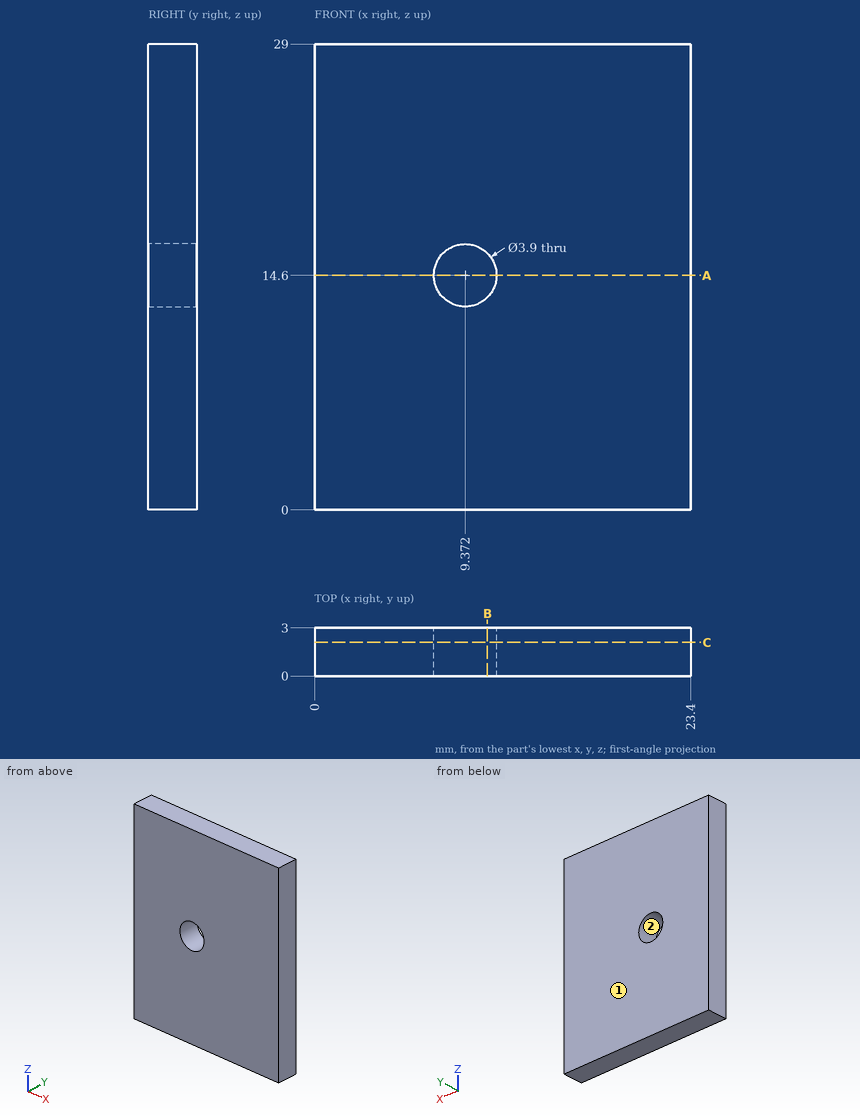
Here's the drawing with two shaded views (mm, measured from the low corner). I have some questions. Give positions to 0.01 mm unless a question says otherwise; leave off trailing zeros. Order: outer loops, then holes, each group sorted by start corner. A loop starts at its lowest first (then second) coordinate and runs counter-clockwise, first axis right, second up.
Q1. If I drill on line 1 along X through (y, z) = (1.95, 14.6); line 2 along X through (y, z) = (1.2, 13); line 3 along Z through (x, y) = (8.25, 0.7) (1 decimal), over which ranges is the centre line in solid material (lowest first)?
Q2. We'd pull the mould along Z, two halves only. Please class the marked faces 1 and 2: +Z half, -Z half, draft (parallel to the pull), parting line (faces both ways), or undercut.
Q3. Suppose I cut it at A-A, the plane z = 14.6. Write out the boundary of the cut face in (x, y).
Q4. Suppose I cut it at B-B, the plane x = 10.75. Write out the boundary of the cut face in (y, z), and give its area (3 significant figures).
Q5. Suppose I cut it at C-C, the plane y = 2.1. Write out the boundary of the cut face in (x, z).
Q6. I'm going to push flat-ended pins straight in: P1, Ø4, axis at x = 5.5, z = 7, coming from the -Y side; P2, Ø3.5, axis at x = 9.37, z = 14.6, coming from the -Y side. Where does each tip first touch, or does it pass through?
Solution:
1. line 1: x = 0 to 7.42, 11.32 to 23.4
1. line 2: x = 0 to 8.26, 10.49 to 23.4
1. line 3: z = 0 to 13, 16.2 to 29
2. face 1: draft
2. face 2: undercut
3. outline: (0, 0) - (7.42, 0) - (7.42, 3) - (0, 3) - close; (11.32, 0) - (23.4, 0) - (23.4, 3) - (11.32, 3) - close
4. outline: (0, 0) - (3, 0) - (3, 13.22) - (0, 13.22) - close; (0, 15.98) - (3, 15.98) - (3, 29) - (0, 29) - close
4. area: 78.7 mm2
5. outline: (0, 0) - (23.4, 0) - (23.4, 29) - (0, 29) - close; hole circle Ø3.9 at (9.37, 14.6)
6. P1: stops at y = 0
6. P2: passes through
